CAD build for the part. Positions are in the model's coordinates, mm. A direction names the side the tool comes from. Coordinates: 2 decimals unless noted, no trailing zeros. Loops run counter-clockwise (first coordinate to the right, second up) from the corner with the lowest first, then second, coordinate; pieces in that order, holes last. Notation, with made-up numbers: (74, 10) -> (82, 10) arc R32 ccw to (82, 36) -> close; hole circle Ø7 at (-7, 64). An arc over 180 degrees is marked (long way). Write item = value, one per line. Start each with the question number.
(1) Band-saw the part on B-B (y = -87). Write the cut outline in (x, z), and give its area (3 significant figures).
(2) Drill centre lines: line 1 (X direction, y = -98, z = -4.5); line 2 (Z direction, x = -1.5, y = -93); line 3 (Z direction, x = 0.25, y = -35). Where is each one in solid material? Low to high. Write a range as from..to.
(3) Flat gauge pins, fed straight in: P1, Ø1.7, axis at x = -4.5, y = -8, coming from the +Z side; P2, Ø1.3, axis at x = 1, y = -85.5, coming from the -Z side; P3, Ø1.9, axis at x = -2, z = 95, coming from the -Y side. Where does each tip first touch, or does it go through?
(4) Tool access for faces 1 (the face through (-4, -101.6, 94)), 2 (the face through (-4, -58.738, 94)), 3 (the face through (-2, -45, 95.374)), 4 (the face through (-2, -88, 98.549)), 5 (the face through (1.493, -88, 94)): list every direction of +Z, -Z, +X, -X, +Y, -Y with a clear straight run to the whole face (end or side of a thin tool).
(5) Pull direction X, two halves, no side cores. Call faces 6 (the face through (1.493, -45, 94)), 7 (the face through (-4, -31.75, 94)), 8 (the face through (-4.857, -68, 41)), 9 (the face through (-2, -88, 95.374)): +X half, -X half, draft (parallel to the pull), parting line (faces both ways), or undercut.
(6) Band-saw the part on A-A (x = -2). Write the cut outline in (y, z), and give its area (3 significant figures).
(7) Band-saw the part on C-C (z = 9.5). Write the cut outline in (x, y), and give its area (3 significant figures).
(8) Band-saw the part on D-D (y = -10.5). Write the cut outline in (x, z).
```python
from build123d import *

# Parameters (mm, degrees)
F0_W     = 1.5875
F0_H     = 12.7
F0_H_2   = 6.35
F0_H_3   = 101.6
F1_DEPTH = 66.675
F3_DEPTH = 7.9375
F5_DEPTH = 31.75


with BuildPart() as f1:
    # F0 (on Front) → F1 (new body)
    with BuildSketch(Plane.XZ):
        Polygon((-4.8573001859, 98.5494344607), (-4.8573001859, 95.3744344607), (-3.2698001859, 95.3744344607), (-0.0948001859, 95.3744344607), (1.4926998141, 95.3744344607), (1.4926998141, 98.5494344607), align=None)
        with Locations((-4.0635501859, 89.0244344607)):
            Rectangle(F0_W, F0_H)
        with Locations((0.6989498141, 92.1994344607)):
            Rectangle(F0_W, F0_H_2)
        with Locations((-4.0635501859, 31.8744344607)):
            Rectangle(F0_W, F0_H_3)
    extrude(amount=F1_DEPTH)

    # F2 (on face) → F3 (cut)
    with BuildSketch(Plane.XZ.offset(66.675)):
        Polygon((-4.8573001859, 98.5494344607), (-4.8573001859, 85.8803465962), (-3.2698001859, 85.8803465962), (-3.2698001859, 95.3744344607), (-0.0948001859, 95.3744344607), (-0.0948001859, 89.0244344607), (1.4926998141, 89.0244344607), (1.4926998141, 98.5494344607), align=None)
    extrude(amount=-F3_DEPTH, mode=Mode.SUBTRACT)

    # F4 (on face) → F5 (cut)
    with BuildSketch(Plane(origin=(0, 0, 0), x_dir=(-1, 0, 0), z_dir=(0, 1, 0))):
        Polygon((3.2698001859, 85.861839354), (4.8573001859, 85.861839354), (4.8573001859, 98.5494344607), (-1.4926998141, 98.5494344607), (-1.4926998141, 89.0244344607), (0.0948001859, 89.0244344607), (0.0948001859, 95.3744344607), (3.2698001859, 95.3744344607), align=None)
    extrude(amount=-F5_DEPTH, mode=Mode.SUBTRACT)

    # F6: F1 across face


with BuildPart() as f1_1:
    add(f1.part)
    add(f1.part.mirror(Plane(origin=(-4.0635501859, -66.675, 33.4773905285), x_dir=(1, 0, 0), z_dir=(0, -1, 0))))


solid = f1_1.part
```
Findings below:
q1.outline = (-4.86, -18.93) -> (-3.27, -18.93) -> (-3.27, 95.37) -> (-0.09, 95.37) -> (-0.09, 89.02) -> (1.49, 89.02) -> (1.49, 98.55) -> (-4.86, 98.55) -> close
q1.area = 212 mm²
q2.line_1 = -4.86..-3.27
q2.line_2 = 95.37..98.55
q2.line_3 = 89.02..98.55
q3.P1 = 85.86
q3.P2 = 89.02
q3.P3 = -101.6
q4.face_1 = +Z, +X, -X, -Y
q4.face_2 = +Z, +X, -X
q4.face_3 = -Z, +Y, -Y
q4.face_4 = +Z, +X, -X, +Y, -Y
q4.face_5 = +Z, -Z, +X, +Y, -Y
q5.face_6 = +X half
q5.face_7 = draft
q5.face_8 = -X half
q5.face_9 = undercut
q6.outline = (-101.6, 95.37) -> (-74.61, 95.37) -> (-74.61, 98.55) -> (-101.6, 98.55) -> close; (-58.74, 95.37) -> (-31.75, 95.37) -> (-31.75, 98.55) -> (-58.74, 98.55) -> close
q6.area = 171 mm²
q7.outline = (-4.86, -133.35) -> (-3.27, -133.35) -> (-3.27, 0) -> (-4.86, 0) -> close
q7.area = 212 mm²
q8.outline = (-4.86, -18.93) -> (-3.27, -18.93) -> (-3.27, 85.86) -> (-4.86, 85.86) -> close
